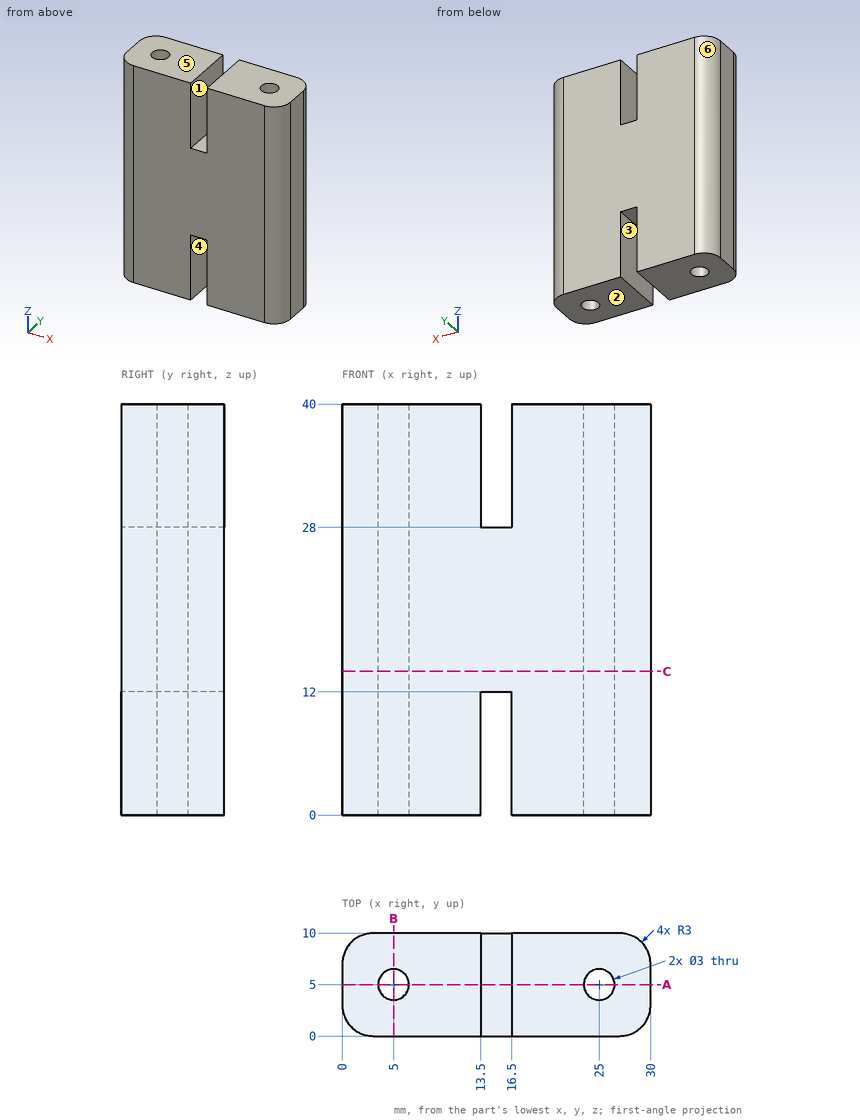
Can you work these out from the drawing? Everything is in mm from the part's minimum corner. A direction names the side the tool comes from. Give positions to 0.01 mm unless a question says otherwise; leave off trailing zeros. Order: outer loops, then holes, each group sorted by start corner. A loop starts at its lowest first (then second) coordinate and runs counter-clockwise, first axis right, second up. Notation, with made-up numbers: M -28,4 L -4,4 A15 cw -4,11 Z; hole C 74.25,80 d2. An arc over 180 degrees is marked long. One line per item, written item: value.
Item 1: If we section it at C-C on z = 14: Write out the boundary of the cut face in (x, y), and give its area (3 significant figures).
Verdict:
outline: M 0,3 A3 ccw 3,0 L 27,0 A3 ccw 30,3 L 30,7 A3 ccw 27,10 L 3,10 A3 ccw 0,7 Z; hole C 5,5 d3; hole C 25,5 d3
area: 278 mm2
Item 2: If we mould it in two halves opening along X, with no side actions, what happens to the marked faces 4, 5 and 6? For each: pulls with the +X half, pulls with the -X half, needs draft (parallel to the pull), parting line crosses it, or undercut.
Verdict:
face 4: undercut
face 5: needs draft
face 6: pulls with the -X half
Item 3: For the marked faces 1, 2 and 3, which set-ups out of +Z, -Z, +X, -X, +Y, -Y let a thin tool reach every point of the face, with its end or its side?
Verdict:
face 1: +Z, +Y, -Y
face 2: -Z, +X, -X, +Y, -Y
face 3: -Z, +Y, -Y
Item 4: If we section it at A-A on y = 5: Write out the boundary of the cut face in (x, z).
Verdict:
outline: M 0,0 L 3.5,0 L 3.5,40 L 0,40 Z; M 6.5,0 L 13.5,0 L 13.5,12 L 16.5,12 L 16.5,0 L 23.5,0 L 23.5,40 L 16.5,40 L 16.5,28 L 13.5,28 L 13.5,40 L 6.5,40 Z; M 26.5,0 L 30,0 L 30,40 L 26.5,40 Z
Item 5: If we section it at B-B on x = 5: Write out the boundary of the cut face in (y, z).
Verdict:
outline: M 0,0 L 3.5,0 L 3.5,40 L 0,40 Z; M 6.5,0 L 10,0 L 10,40 L 6.5,40 Z
Item 6: For pin 1 (1.5 mm diameter, centred on y = 8, z = 17.5, fed in from +X); pin 2 (2.5 mm diameter, centred on x = 5, y = 5, fed in from +Z), each with a flat end and sliding along its axis, tell me the tip position at first contact or that it passes through.
Verdict:
pin 1: x = 29.99
pin 2: through
Item 7: Please list where these lines run through material, in increasing order: line 1 (Y direction, x = 25, z = 31); line 2 (X direction, y = 4.75, z = 14.5); line 3 (X direction, y = 6, z = 19).
Verdict:
line 1: 0 to 3.5, 6.5 to 10
line 2: 0 to 3.52, 6.48 to 23.52, 26.48 to 30
line 3: 0 to 3.88, 6.12 to 23.88, 26.12 to 30
